```python
from build123d import *

# Parameters (mm, degrees)
F0_W     = 35.2
F0_H     = 35.2
F1_DEPTH = 52
F2_SIZE  = 3
F3_R     = 11
F4_DEPTH = 2
F5_R     = 2.5
F6_DEPTH = 24
F7_R     = 1.5
F8_DEPTH = 10


# Not quite as in the source:
# - a feature names something its author has since deleted; it is built from what else it names


with BuildPart() as f1:
    # F0 (on Top) → F1 (new body)
    with BuildSketch(Plane.XY):
        with Locations((17.6, 17.6)):
            Rectangle(F0_W, F0_H)
    extrude(amount=F1_DEPTH)

    # F2
    f2_edges = [f1.edges().sort_by_distance(p)[0] for p in [
        (0, 0, 26),
        (0, 35.2, 26),
        (35.2, 0, 26),
        (35.2, 35.2, 26),
    ]]
    chamfer(f2_edges, length=F2_SIZE)

    # F3 (on face) → F4 (join)
    with BuildSketch(Plane.XY.offset(52)):
        with Locations((17.6, 17.6)):
            Circle(F3_R)
    extrude(amount=F4_DEPTH)

    # F5 (on face) → F6 (join)
    with BuildSketch(Plane.XY.offset(54)):
        with Locations((17.6, 17.6)):
            Circle(F5_R)
    extrude(amount=F6_DEPTH)

    # F7 (on face) → F8 (cut)
    with BuildSketch(Plane.XY.offset(52)):
        with Locations((4.6, 30.6)):
            Circle(F7_R)
        with Locations((4.6, 4.6)):
            Circle(F7_R)
        with Locations((30.6, 30.6)):
            Circle(F7_R)
        with Locations((30.6, 4.6)):
            Circle(F7_R)
    extrude(amount=-F8_DEPTH, mode=Mode.SUBTRACT)


solid = f1.part
```
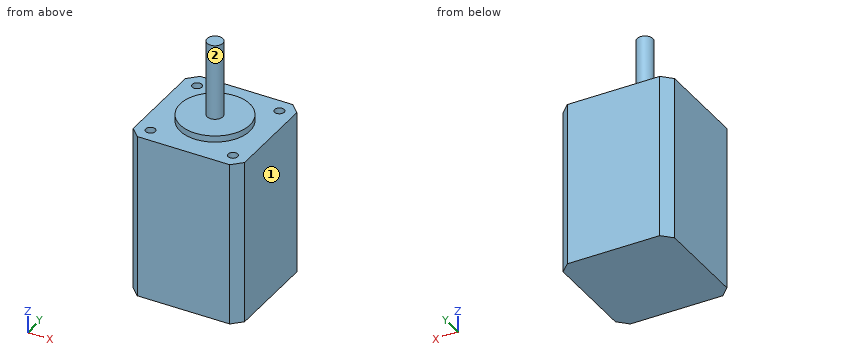
Source: CAD feature listing. Evaluate the final solid. Frame: model axes, mm. Face numbers are marked on the shaded views. A direction names the side the tool comes from. Round coordinates to 2 decimals unless told otherwise and drop trailing zeros. Write each loop counter-clockwise with the first axis right and the second up, starting at its lowest first coordinate (ties: lowest second). Pieces come first, ordered by that corner, then holes. Notation, with made-up numbers: M 60,39 L 103,39 A25 ccw 103,57 Z; hole C 56.5,15.5 d7. An arc over 180 degrees is marked long. Use CSV: the item, a comma, the result in double quotes. Start each with the question number.
Q1. Line query: line 1 (Y direction, x = 4.6, z = 44); line 2 (X direction, y = 4, z = 45); line 3 (Y direction, x = 31, z = 47). Output: solid intervals per line, ascending. Write a range as from..to.
Q2. Cut plane A-A on x = 17.6. Output: boundary loops of the cut face in (y, z).
Q3. Cut plane D-D on y = 21.5. Output: boundary loops of the cut face in (x, z), plus the area to 3 significant figures.
Q4. First-contact query: P1, Ø5, axis at x = 30.6, y = 30.6, coming from the -Z side; P2, Ø1.5, axis at x = 4, y = 4.5, coming from the +Z side; P3, Ø3.5, axis at x = 31, y = 4, coming from the +Z side. Flat tips, straight axial feed; report the tip coordinate or a pass-through.
Q5. Cut plane C-C on z = 64.5. Output: boundary loops of the cut face in (x, y).
Q6. Cut plane B-B on y = 30.6. Output: boundary loops of the cut face in (x, z).
Q7. Access query for the marked faces 1 and 2. Directions: +Z, -Z, +X, -X, +Y, -Y. A direction counts if a zero-diameter tool reaches every point of the face in a straight line with its end or side. Return the directions, or none.
Results found:
1,line 1,"0..3.1, 6.1..29.1, 32.1..35.2"
1,line 2,"0..3.23, 5.97..29.23, 31.97..35.2"
1,line 3,"0..3.15, 6.05..29.15, 32.05..35.2"
2,outline,"M 0,0 L 35.2,0 L 35.2,52 L 28.6,52 L 28.6,54 L 20.1,54 L 20.1,78 L 15.1,78 L 15.1,54 L 6.6,54 L 6.6,52 L 0,52 Z"
3,outline,"M 0,0 L 35.2,0 L 35.2,52 L 27.89,52 L 27.89,54 L 7.31,54 L 7.31,52 L 0,52 Z"
3,area,"1,870 mm^2"
4,P1,"z = 0"
4,P2,"z = 42"
4,P3,"z = 52"
5,outline,"C 17.6,17.6 d5"
6,outline,"M 0,0 L 35.2,0 L 35.2,52 L 32.1,52 L 32.1,42 L 29.1,42 L 29.1,52 L 6.1,52 L 6.1,42 L 3.1,42 L 3.1,52 L 0,52 Z"
7,face 1,"+Z, -Z, +X, +Y, -Y"
7,face 2,"+Z"
